Geometry check sheet. Reference: the model listing, model coordinates, mm. Face numbers are marked on the shaded views. Coordinates: 2 decimals unless noted, no trailing zeros. Order: outer loops, then holes, each group sorted by start corner. A loop starts at its lowest first (then second) coordinate and runs counter-clockwise, first axis right, second up.
```python
from build123d import *

# Parameters (mm, degrees)
F0_R     = 11
F1_DEPTH = 8


with BuildPart() as f1:
    # F0 (on Top) → F1 (new body)
    with BuildSketch(Plane.XY):
        with BuildLine():
            ThreePointArc((-9.6073463611, 24.6428649543), (-2.7675973359, 40.6461450763), (11, 30))
            ThreePointArc((11, 30), (10.6461450763, 27.2324026641), (9.6073463611, 24.6428649543))
            add(Edge.make_bspline(
                [(9.6073463611, 24.6428649543), (14.4035735746, 25.6322402973), (18.3329413126, 27.4179519792), (20, 30)],
                knots=[0.8849975762, 0.8849975762, 0.8849975762, 0.8849975762, 1, 1, 1, 1], degree=3))
            add(Edge.make_bspline(
                [(20, 30), (24.5452855367, 37.0400314114), (0, 62.9599685886), (-24.5452855367, 37.0400314114), (-20, 30)],
                knots=[0, 0, 0, 0, 0.3135575596, 0.6271151192, 0.6271151192, 0.6271151192, 0.6271151192], degree=3))
            add(Edge.make_bspline(
                [(-20, 30), (-18.3329413126, 27.4179519792), (-14.4035735746, 25.6322402973), (-9.6073463611, 24.6428649543)],
                knots=[0.6271151192, 0.6271151192, 0.6271151192, 0.6271151192, 0.742117543, 0.742117543, 0.742117543, 0.742117543], degree=3))
        make_face()
        with BuildLine():
            ThreePointArc((9.6073463611, 24.6428649543), (0, 19), (-9.6073463611, 24.6428649543))
            add(Edge.make_bspline(
                [(-20, 30), (-18.3329413126, 27.4179519792), (-14.4035735746, 25.6322402973), (-9.6073463611, 24.6428649543)],
                knots=[0.6271151192, 0.6271151192, 0.6271151192, 0.6271151192, 0.742117543, 0.742117543, 0.742117543, 0.742117543], degree=3))
            ThreePointArc((-20, 30), (-14.161984871, 0), (-20, -30))
            add(Edge.make_bspline(
                [(-20, -30), (-18.3329413126, -27.4179519792), (-14.4035735746, -25.6322402973), (-9.6073463611, -24.6428649543)],
                knots=[0.6271151192, 0.6271151192, 0.6271151192, 0.6271151192, 0.742117543, 0.742117543, 0.742117543, 0.742117543], degree=3))
            ThreePointArc((-9.6073463611, -24.6428649543), (0, -19), (9.6073463611, -24.6428649543))
            add(Edge.make_bspline(
                [(9.6073463611, -24.6428649543), (14.4035735746, -25.6322402973), (18.3329413126, -27.4179519792), (20, -30)],
                knots=[0.8849975762, 0.8849975762, 0.8849975762, 0.8849975762, 1, 1, 1, 1], degree=3))
            ThreePointArc((20, -30), (14.161984871, 0), (20, 30))
            add(Edge.make_bspline(
                [(9.6073463611, 24.6428649543), (14.4035735746, 25.6322402973), (18.3329413126, 27.4179519792), (20, 30)],
                knots=[0.8849975762, 0.8849975762, 0.8849975762, 0.8849975762, 1, 1, 1, 1], degree=3))
        make_face()
        Circle(F0_R, mode=Mode.SUBTRACT)
        with BuildLine():
            add(Edge.make_bspline(
                [(-20, -30), (-18.3329413126, -27.4179519792), (-14.4035735746, -25.6322402973), (-9.6073463611, -24.6428649543)],
                knots=[0.6271151192, 0.6271151192, 0.6271151192, 0.6271151192, 0.742117543, 0.742117543, 0.742117543, 0.742117543], degree=3))
            add(Edge.make_bspline(
                [(20, -30), (24.5452855367, -37.0400314114), (0, -62.9599685886), (-24.5452855367, -37.0400314114), (-20, -30)],
                knots=[0, 0, 0, 0, 0.3135575596, 0.6271151192, 0.6271151192, 0.6271151192, 0.6271151192], degree=3))
            add(Edge.make_bspline(
                [(9.6073463611, -24.6428649543), (14.4035735746, -25.6322402973), (18.3329413126, -27.4179519792), (20, -30)],
                knots=[0.8849975762, 0.8849975762, 0.8849975762, 0.8849975762, 1, 1, 1, 1], degree=3))
            ThreePointArc((9.6073463611, -24.6428649543), (10.6461450763, -27.2324026641), (11, -30))
            ThreePointArc((11, -30), (-2.7675973359, -40.6461450763), (-9.6073463611, -24.6428649543))
        make_face()
    extrude(amount=F1_DEPTH)


solid = f1.part
```
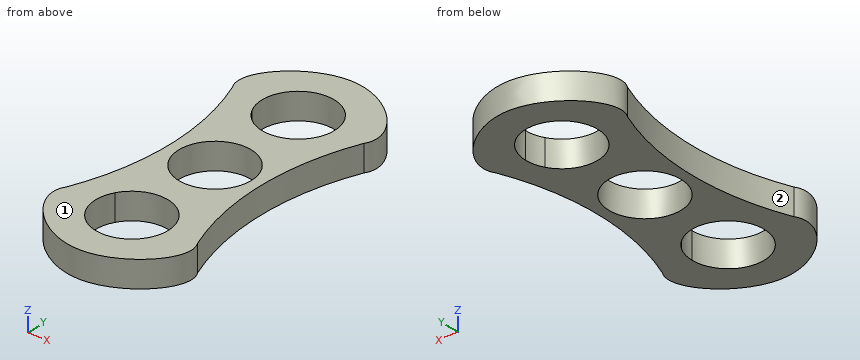
Item 1: Sectioned sample at D-D (y = 26). Record the cut outline in (x, z), and give its area (3 significant figures).
Item 2: Sectioned sample at A-A (y = 0). Record the cut outline in (x, z).
Item 3: Sectioned sample at B-B (x = 0). Give the number of separate pieces and of enclosed holes in the cut face, and give its area (3 significant figures).
Item 4: Release check for a two-part mould opening along Y. For the marked faces 1 and 2 record: pulls with the +Y half, pulls with the -Y half, needs draft (parallel to the pull), parting line crosses it, or undercut.
Item 5: Thickness scan on line 1 along Y through (x, z) = (0, 5.25); line 2 along Y through (x, z) = (5, 3.75); line 3 along X through (y, z) = (-30, 2). Record the ranges inside material, lowest first.
Item 6: Depth check by flat-ended pin: P1, Ø3, axis at x = -10, y = 2, coming from the -Z side; P2, Ø2, axis at y = 10.5, z = 3, coming from the +X side; P3, Ø1.5, axis at x = -1.5, z = 6.5, coming from the +Y side. Enter the tip coordinate at first touch or a pass-through.
Geometry check:
1. outline: (-18.5, 0) - (-10.25, 0) - (-10.25, 8) - (-18.5, 8) - close; (10.25, 0) - (18.5, 0) - (18.5, 8) - (10.25, 8) - close
1. area: 132 mm2
2. outline: (-14.16, 0) - (-11, 0) - (-11, 8) - (-14.16, 8) - close; (11, 0) - (14.16, 0) - (14.16, 8) - (11, 8) - close
3. separate pieces: 4
3. enclosed holes: 0
3. area: 272 mm2
4. face 1: needs draft
4. face 2: undercut
5. line 1: y = -50 to -41, -19 to -11, 11 to 19, 41 to 50
5. line 2: y = -49.32 to -39.8, -20.2 to -9.8, 9.8 to 20.2, 39.8 to 49.32
5. line 3: x = -20 to -11, 11 to 20
6. P1: stops at z = 0
6. P2: stops at x = 14.99
6. P3: stops at y = 49.98
